Geometry check sheet. Reference: drawing and pictorial views, mm from the part's lowest x, y, z. Coordinates: 2 decimals unless noted, no trailing zeros. Write each loop counter-clockwise with the first axis right and the second up, starting at its lowest first coordinate (ties: lowest second). Pieces come first, ordered by that corner, then holes. Notation, with made-up numbers: M 28,-30 L 78,-30 A30 ccw 78,-5 Z; hole C -22.75,22.25 d6. An arc over 180 degrees is marked long. One line per item, written item: value.
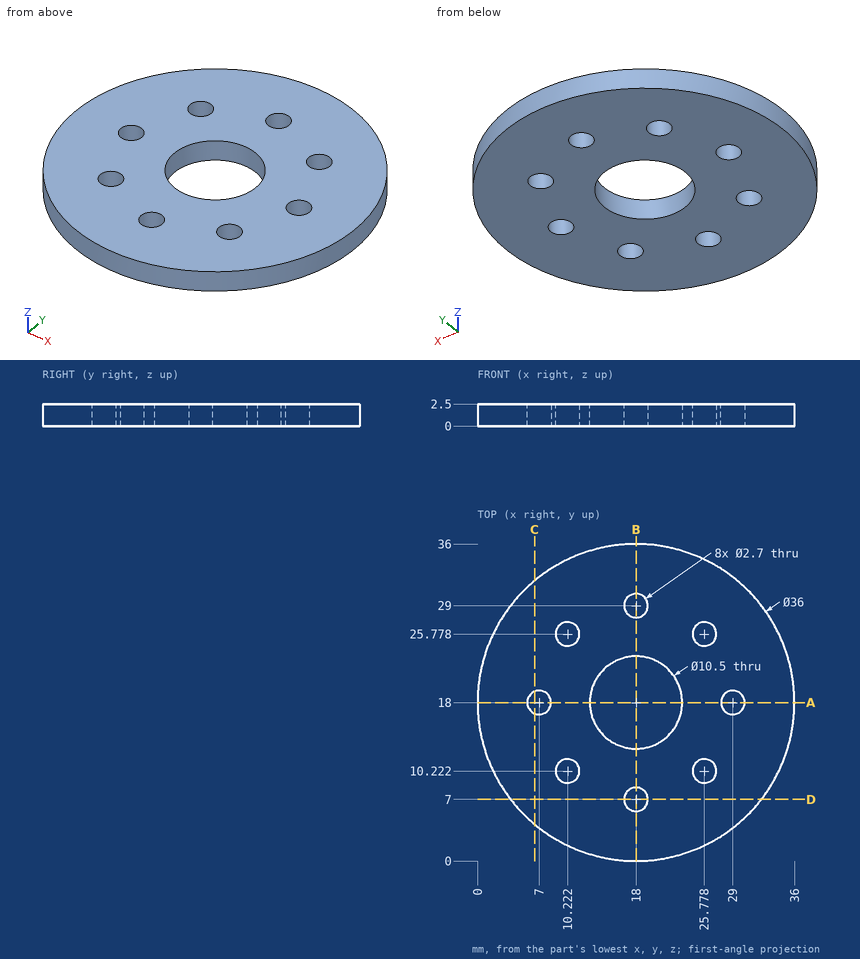
Item 1: Cross-section at A-A, the plane y = 18. Enter the section's corners in (x, z).
The answers:
outline: M 0,0 L 5.65,0 L 5.65,2.5 L 0,2.5 Z; M 8.35,0 L 12.75,0 L 12.75,2.5 L 8.35,2.5 Z; M 23.25,0 L 27.65,0 L 27.65,2.5 L 23.25,2.5 Z; M 30.35,0 L 36,0 L 36,2.5 L 30.35,2.5 Z
Item 2: Cross-section at D-D, the plane y = 7. Enter the section's corners in (x, z), and give its area (3 significant figures).
The answers:
outline: M 3.75,0 L 16.65,0 L 16.65,2.5 L 3.75,2.5 Z; M 19.35,0 L 32.25,0 L 32.25,2.5 L 19.35,2.5 Z
area: 64.5 mm²
Item 3: Go/stop test with flat-tipped pins: P1, Ø2, axis at x = 18, y = 7, coming from the +Z side; P2, Ø1, axis at x = 6, z = 2, coming from the -Y side. Record where each tip stops, or that it passes through.
The answers:
P1: passes through
P2: stops at y = 4.15
Item 4: Scan lines: line 1 (Y direction, x = 18, z = 0.75); line 2 (X direction, y = 9.5, z = 0.25). Record each from-to range of solid material in increasing order.
The answers:
line 1: y = 0 to 5.65, 8.35 to 12.75, 23.25 to 27.65, 30.35 to 36
line 2: x = 2.13 to 9.08, 11.36 to 24.64, 26.92 to 33.87
Item 5: Cross-section at C-C, the plane x = 6.5. Enter the section's corners in (y, z).
The answers:
outline: M 4.15,0 L 16.75,0 L 16.75,2.5 L 4.15,2.5 Z; M 19.25,0 L 31.85,0 L 31.85,2.5 L 19.25,2.5 Z
